Verification items for this drawing (mm, ordinates from the low corner). Round coordinates to 2 decimals unless told otherwise and drop trailing zeros. Order: outer loops, then holes, each group sorted by start corner. A loop starts at its lowest first (then second) coordinate and runs counter-clockwise, first axis right, second up. Notation, with made-up numbers: M 6,65.5 L 21,65.5 A18 ccw 21,94.5 Z; hole C 18.25,-28 d2. An arc over 180 degrees is marked long. One line per item, written item: value. Start each with the question number.
(1) Cross-section at B-B, the plane y = 1.7. Enter the section's corners in (x, z), and give its area (3 significant figures).
(2) Depth check by flat-ended pin: pin 1 Ø2 at (x, y) = (109, 1) entering from -Z. Enter the tip coordinate at first touch or a pass-through.
(3) Thickness scan on L1, parallel to Z at x = 102.5, y = 1.5; L2, parallel to X at y = 2.9, z = 71; L3, parallel to X at y = 0.35, z = 22. Record the ranges inside material, lowest first.
(4) Cross-section at A-A, the plane z = 26. Enter the section's corners in (x, y).
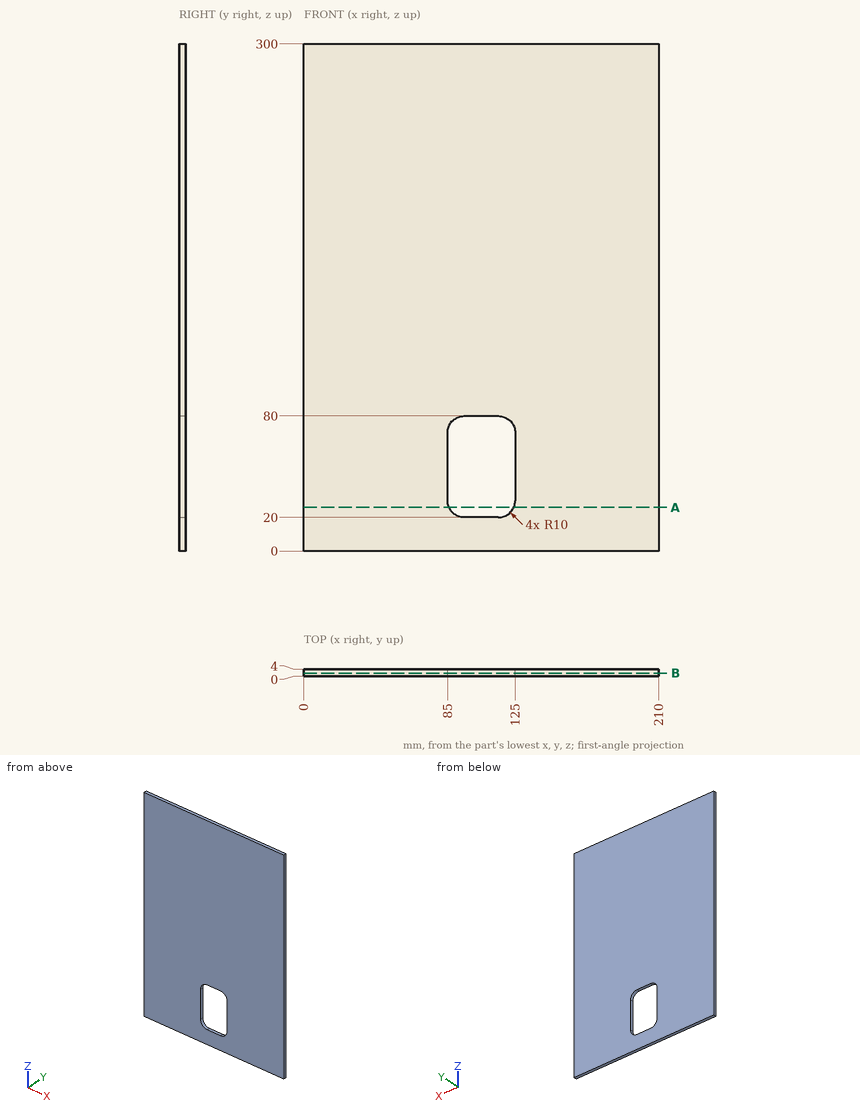
Values found:
1. outline: M 0,0 L 210,0 L 210,300 L 0,300 Z; hole M 85,30 A10 ccw 95,20 L 115,20 A10 ccw 125,30 L 125,70 A10 ccw 115,80 L 95,80 A10 ccw 85,70 Z
1. area: 60,700 mm^2
2. pin 1: z = 0
3. L1: 0 to 20, 80 to 300
3. L2: 0 to 85.05, 124.95 to 210
3. L3: 0 to 89, 121 to 210
4. outline: M 0,0 L 85.83,0 L 85.83,4 L 0,4 Z; M 124.17,0 L 210,0 L 210,4 L 124.17,4 Z
